from build123d import *

# Parameters (mm, degrees)
BOSS_EXTRUDE1_DEPTH     = 19.05
CUT_EXTRUDE1_DEPTH      = 14.1224
CUT_EXTRUDE2_DEPTH      = 52.976990101
CUT_EXTRUDE2_DEPTH_BACK = 52.976990101
SKETCH4_R               = 2.38125
CUT_EXTRUDE3_DEPTH      = 52.976990138
CUT_EXTRUDE3_DEPTH_BACK = 52.976990138
SKETCH5_R               = 2.38125
CUT_EXTRUDE4_DEPTH      = 52.97699026
CUT_EXTRUDE4_DEPTH_BACK = 52.97699026
SKETCH7_R               = 2.38125


with BuildPart() as part:
    # Sketch2 → Boss-Extrude1 (new body)
    with BuildSketch(Plane.XY):
        with BuildLine():
            Line((3.175, 0), (41.275, 0))
            ThreePointArc((41.275, 0), (43.52006403, 0.92993597), (44.45, 3.175))
            Line((44.45, 3.175), (44.45, 15.875))
            ThreePointArc((44.45, 15.875), (43.52006403, 18.12006403), (41.275, 19.05))
            Line((41.275, 19.05), (3.175, 19.05))
            ThreePointArc((3.175, 19.05), (0.92993597, 18.12006403), (0, 15.875))
            Line((0, 15.875), (0, 3.175))
            ThreePointArc((0, 3.175), (0.92993597, 0.92993597), (3.175, 0))
        make_face()
    extrude(amount=BOSS_EXTRUDE1_DEPTH)

    # Sketch3 → Cut-Extrude1 (cut)
    with BuildSketch(Plane(origin=(0, 0, 0), x_dir=(-1, 0, 0), z_dir=(0, 0, -1))):
        with BuildLine():
            Line((-34.925, 14.2875), (-9.525, 14.2875))
            ThreePointArc((-9.525, 14.2875), (-4.7625, 9.525), (-9.525, 4.7625))
            Line((-9.525, 4.7625), (-34.925, 4.7625))
            ThreePointArc((-34.925, 4.7625), (-39.6875, 9.525), (-34.925, 14.2875))
        make_face()
    extrude(amount=-CUT_EXTRUDE1_DEPTH, mode=Mode.SUBTRACT)

    # Sketch4 → Cut-Extrude2 (cut, two sides: drawn at the far end of the back side and taken through both)
    with BuildSketch(Plane(origin=(0, 19.05, 0), x_dir=(1, 0, 0), z_dir=(0, 1, 0)).offset(-CUT_EXTRUDE2_DEPTH_BACK)):
        with Locations(Location((34.925, -6.35, 0), (0, 0, 270))):
            Circle(SKETCH4_R)
        with Locations(Location((22.225, -6.35, 0), (0, 0, 270))):
            Circle(SKETCH4_R)
        with Locations(Location((9.525, -6.35, 0), (0, 0, 270))):
            Circle(SKETCH4_R)
    extrude(amount=CUT_EXTRUDE2_DEPTH + CUT_EXTRUDE2_DEPTH_BACK, mode=Mode.SUBTRACT)

    # Sketch5 → Cut-Extrude3 (cut, two sides: drawn at the far end of the back side and taken through both)
    with BuildSketch(Plane(origin=(44.45, 0, 0), x_dir=(0, 0, -1), z_dir=(1, 0, 0)).offset(-CUT_EXTRUDE3_DEPTH_BACK)):
        with Locations((-6.35, 9.525)):
            Circle(SKETCH5_R)
    extrude(amount=CUT_EXTRUDE3_DEPTH + CUT_EXTRUDE3_DEPTH_BACK, mode=Mode.SUBTRACT)

    # Sketch7 → Cut-Extrude4 (cut, two sides: drawn at the far end of the back side and taken through both)
    with BuildSketch(Plane.XY.offset(19.05).offset(-CUT_EXTRUDE4_DEPTH_BACK)):
        with Locations((22.225, 9.525)):
            Circle(SKETCH7_R)
        with Locations((34.925, 9.525)):
            Circle(SKETCH7_R)
        with Locations((9.525, 9.525)):
            Circle(SKETCH7_R)
    extrude(amount=CUT_EXTRUDE4_DEPTH + CUT_EXTRUDE4_DEPTH_BACK, mode=Mode.SUBTRACT)


solid = part.part
Build history of the part. All positions in model axes, mm. A direction names the side the tool comes from. Give positions to 0.01 mm unless a question says otherwise; leave off trailing zeros. Loops run counter-clockwise (first coordinate to the right, second up) from the corner with the lowest first, then second, coordinate; pieces in that order, holes last. Notation, with made-up numbers: (-32.5, 61) - (-4.5, 61) arc R10 ccw to (-4.5, 71) - close; hole circle Ø6 at (36, 58). An arc over 180 degrees is marked (long way). Write item = value, one per line. Start each with the question number.
1) Drop flat-ended pins along their axis: pin 1 Ø3 at (x, z) = (11, 7.5) entering from -Y; pin 2 Ø3 at (x, y) = (20.5, 9.5) entering from -Z. Give the stop position or say it passes through.
2) Tool access for faces 4 (the cylindrical face through (19.9, 2.35, 5.83)), 5 (the cylindrical face through (5.015, 7.995, 8.531)): list every direction of +Z, -Z, +X, -X, +Y, -Y with a clear straight run to the whole face (end or side of a thin tool).
3) Pull direction Z, two halves, no side cores. Call faces 1 (the flat face through (22, 13, 14.122)), 2 (the cylindrical face through (2.66, 10.24, 4.08)), 3 (the cylindrical face through (43.5, 0.91, 9.39)): +Z half, -Z half, draft (parallel to the pull), parting line (faces both ways), or undercut.
4) Band-saw the part on D-D on x = 33. Give the cut face in (y, z).
5) Band-saw the part on B-B on x = 26.5. Give the cut face in (y, z), plus the area to 3 significant figures.
6) Band-saw the part on C-C on y = 11. Give the cut face in (x, z), plus the area to 3 significant figures.
7) Probe probe 1 along Y at (x, z) = (19, 6.25); probe 2 along X at (y, z) = (18, 6.35); probe 3 along X at (y, z) = (18.5, 5.25). List the from-to ranges inside material, lowest first. Write a range as from..to.
Final values:
q1.pin_1 = 0
q1.pin_2 = 14.12
q2.face_4 = +Y, -Y
q2.face_5 = -Z
q3.face_1 = -Z half
q3.face_2 = undercut
q3.face_3 = draft
q4.outline = (0, 0) - (4.76, 0) - (4.76, 4.95) - (0, 4.95) - close; (0, 7.75) - (4.76, 7.75) - (4.76, 14.12) - (8.12, 14.12) - (8.12, 19.05) - (0, 19.05) - close; (10.93, 14.12) - (14.29, 14.12) - (14.29, 7.75) - (19.05, 7.75) - (19.05, 19.05) - (10.93, 19.05) - close; (14.29, 0) - (19.05, 0) - (19.05, 4.95) - (14.29, 4.95) - close
q5.outline = (0, 0) - (4.76, 0) - (4.76, 14.12) - (14.29, 14.12) - (14.29, 0) - (19.05, 0) - (19.05, 19.05) - (0, 19.05) - close
q5.area = 228 mm²
q6.outline = (0, 0) - (5, 0) - (5, 4.48) - (0, 4.48) - close; (0, 8.22) - (5, 8.22) - (5, 14.12) - (7.66, 14.12) - (7.66, 19.05) - (0, 19.05) - close; (11.39, 14.12) - (20.36, 14.12) - (20.36, 19.05) - (11.39, 19.05) - close; (24.09, 14.12) - (33.06, 14.12) - (33.06, 19.05) - (24.09, 19.05) - close; (36.79, 14.12) - (39.45, 14.12) - (39.45, 8.22) - (44.45, 8.22) - (44.45, 19.05) - (36.79, 19.05) - close; (39.45, 0) - (44.45, 0) - (44.45, 4.48) - (39.45, 4.48) - close
q6.area = 268 mm²
q7.probe_1 = 0..4.76, 14.29..19.05
q7.probe_2 = 0.82..7.14, 11.91..19.84, 24.61..32.54, 37.31..43.63
q7.probe_3 = 1.39..7.41, 11.64..20.11, 24.34..32.81, 37.04..43.06
